For this review, use the dimensioned drawing (mm, ordinates from the lowest corner) and the shaded views. Give positions to 0.01 mm unless a question says otherwise; leave off trailing zeros. Order: outer loops, then holes, each group sorted by start corner. A loop starts at its lowest first (then second) coordinate and runs counter-clockwise, first axis right, second up. Notation, with made-up numbers: (7.25, 78) - (57.25, 78) arc R9 cw to (57.25, 88) - close; hole circle Ø6 at (89, -8.5). An arc over 180 degrees is marked (long way). Use a Markdown table: item, result. Add a question column.
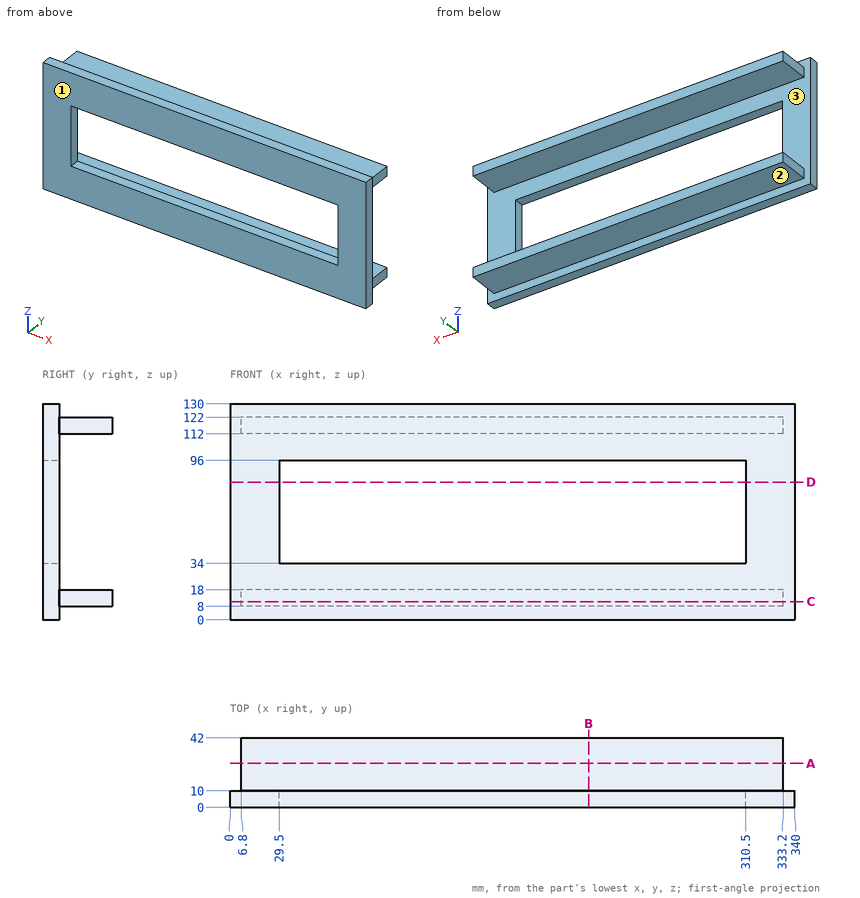
Q1. Draft analysis for pull direction Z (two halves, no side actions). For the marked faces 1, 2 and 3, state which applies: pulls with the +Z half, pulls with the -Z half, needs draft (parallel to the pull), parting line crosses it, or undercut.
Q2. Clearance check with flat-ended pins moving along their axes: P1, Ø5, axis at y = 28, z = 13, coming from the +X side; P2, Ø9.5, axis at x = 247, y = 33, coming from the -Z side; P3, Ø5, axis at y = 23.5, z = 114.5, coming from the -X side. State where each tip first meets the part, or that it passes through.
Q3. Wall thickness on probe 1 along Z at (x, y) = (78, 23); probe 2 along X at (y, z) = (2.5, 92); probe 3 along Z at (x, y) = (82.5, 7.5): over which ranges is each line inside the solid? List them lowest first.
Q4. We need section B-B (x = 216). Write out the cut boundary in (y, z), plus the area to 3 significant figures.
Q5. We need section C-C (z = 11). Write out the cut boundary in (x, y), plus the area to 3 significant figures.
Q6. We need section A-A (y = 26.5). Write out the cut boundary in (x, z), plus the area to 3 significant figures.
Q7. We need section D-D (z = 83). Write out the cut boundary in (x, y), plus the area to 3 significant figures.
Here are the results:
| question | item | result |
|---|---|---|
| 1 | face 1 | needs draft |
| 1 | face 2 | pulls with the -Z half |
| 1 | face 3 | undercut |
| 2 | P1 | x = 333.2 |
| 2 | P2 | z = 8 |
| 2 | P3 | x = 6.8 |
| 3 | probe 1 | 8 to 18, 112 to 122 |
| 3 | probe 2 | 0 to 29.5, 310.5 to 340 |
| 3 | probe 3 | 0 to 34, 96 to 130 |
| 4 | outline | (0, 0) - (10, 0) - (10, 8) - (42, 8) - (42, 18) - (10, 18) - (10, 34) - (0, 34) - close; (0, 96) - (10, 96) - (10, 112) - (42, 112) - (42, 122) - (10, 122) - (10, 130) - (0, 130) - close |
| 4 | area | 1,320 mm2 |
| 5 | outline | (0, 0) - (340, 0) - (340, 10) - (333.2, 10) - (333.2, 42) - (6.8, 42) - (6.8, 10) - (0, 10) - close |
| 5 | area | 13,800 mm2 |
| 6 | outline | (6.8, 8) - (333.2, 8) - (333.2, 18) - (6.8, 18) - close; (6.8, 112) - (333.2, 112) - (333.2, 122) - (6.8, 122) - close |
| 6 | area | 6,530 mm2 |
| 7 | outline | (0, 0) - (29.5, 0) - (29.5, 10) - (0, 10) - close; (310.5, 0) - (340, 0) - (340, 10) - (310.5, 10) - close |
| 7 | area | 590 mm2 |
